Geometry check sheet. Reference: the model listing, model coordinates, mm. Give positions to 0.01 mm unless a question says otherwise; leave off trailing zeros. Loops run counter-clockwise (first coordinate to the right, second up) from the corner with the lowest first, then second, coordinate; pieces in that order, holes last.
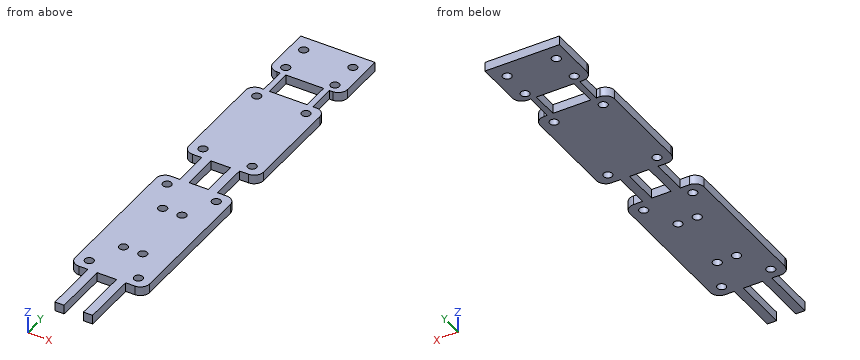
```python
from build123d import *

# Parameters (mm, degrees)
SKETCH1_R           = 0.95
SKETCH1_W           = 4.2
SKETCH1_H           = 8
SKETCH1_W_2         = 8.2
SKETCH1_H_2         = 6
BOSS_EXTRUDE1_DEPTH = 2


with BuildPart() as part:
    # Sketch1 → Boss-Extrude1 (new body)
    with BuildSketch(Plane.XY):
        with BuildLine():
            Line((16.2, 109.64), (0, 109.64))
            Line((0, 109.64), (0, 99.66))
            ThreePointArc((0, 99.66), (0.585786438, 98.245786438), (2, 97.66))
            Line((2, 97.66), (2.75, 97.66))
            Line((2.75, 97.66), (2.75, 91.66))
            Line((2.75, 91.66), (2, 91.66))
            ThreePointArc((2, 91.66), (0.585786438, 91.074213562), (0, 89.66))
            Line((0, 89.66), (0, 69.21))
            ThreePointArc((0, 69.21), (0.585786438, 67.795786438), (2, 67.21))
            Line((2, 67.21), (4, 67.21))
            Line((4, 67.21), (4, 59.21))
            Line((4, 59.21), (2, 59.21))
            ThreePointArc((2, 59.21), (0.585786438, 58.624213562), (0, 57.21))
            Line((0, 57.21), (0, 28))
            ThreePointArc((0, 28), (0.585786438, 26.585786438), (2, 26))
            Line((2, 26), (4, 26))
            Line((4, 26), (4, 14))
            Line((4, 14), (6, 14))
            Line((6, 14), (6, 26))
            Line((6, 26), (10.2, 26))
            Line((10.2, 26), (10.2, 14))
            Line((10.2, 14), (12.2, 14))
            Line((12.2, 14), (12.2, 26))
            Line((12.2, 26), (14.2, 26))
            ThreePointArc((14.2, 26), (15.614213562, 26.585786438), (16.2, 28))
            Line((16.2, 28), (16.2, 57.21))
            ThreePointArc((16.2, 57.21), (15.614213562, 58.624213562), (14.2, 59.21))
            Line((14.2, 59.21), (12.2, 59.21))
            Line((12.2, 59.21), (12.2, 67.21))
            Line((12.2, 67.21), (14.2, 67.21))
            ThreePointArc((14.2, 67.21), (15.614213562, 67.795786438), (16.2, 69.21))
            Line((16.2, 69.21), (16.2, 89.66))
            ThreePointArc((16.2, 89.66), (15.614213562, 91.074213562), (14.2, 91.66))
            Line((14.2, 91.66), (13.45, 91.66))
            Line((13.45, 91.66), (13.45, 97.66))
            Line((13.45, 97.66), (14.2, 97.66))
            ThreePointArc((14.2, 97.66), (15.614213562, 98.245786438), (16.2, 99.66))
            Line((16.2, 99.66), (16.2, 109.64))
        make_face()
        with Locations((13.45, 56.71)):
            Circle(SKETCH1_R, mode=Mode.SUBTRACT)
        with Locations((10.2, 49.71)):
            Circle(SKETCH1_R, mode=Mode.SUBTRACT)
        with Locations((13.45, 106.16)):
            Circle(SKETCH1_R, mode=Mode.SUBTRACT)
        with Locations((2.75, 99.66)):
            Circle(SKETCH1_R, mode=Mode.SUBTRACT)
        with Locations((6, 49.71)):
            Circle(SKETCH1_R, mode=Mode.SUBTRACT)
        with Locations((2.75, 28.5)):
            Circle(SKETCH1_R, mode=Mode.SUBTRACT)
        with Locations((2.75, 89.16)):
            Circle(SKETCH1_R, mode=Mode.SUBTRACT)
        with Locations((2.75, 56.71)):
            Circle(SKETCH1_R, mode=Mode.SUBTRACT)
        with Locations((13.45, 89.16)):
            Circle(SKETCH1_R, mode=Mode.SUBTRACT)
        with Locations((13.45, 99.66)):
            Circle(SKETCH1_R, mode=Mode.SUBTRACT)
        with Locations((13.45, 69.71)):
            Circle(SKETCH1_R, mode=Mode.SUBTRACT)
        with Locations((6, 35.5)):
            Circle(SKETCH1_R, mode=Mode.SUBTRACT)
        with Locations((2.75, 106.16)):
            Circle(SKETCH1_R, mode=Mode.SUBTRACT)
        with Locations((10.2, 35.5)):
            Circle(SKETCH1_R, mode=Mode.SUBTRACT)
        with Locations((2.75, 69.71)):
            Circle(SKETCH1_R, mode=Mode.SUBTRACT)
        with Locations((13.45, 28.5)):
            Circle(SKETCH1_R, mode=Mode.SUBTRACT)
        with Locations((8.1, 63.21)):
            Rectangle(SKETCH1_W, SKETCH1_H, mode=Mode.SUBTRACT)
        with Locations((8.1, 94.66)):
            Rectangle(SKETCH1_W_2, SKETCH1_H_2, mode=Mode.SUBTRACT)
    extrude(amount=BOSS_EXTRUDE1_DEPTH)


solid = part.part
```
1) Sectioned sample at A-A on y = 96. Enter the section's corners in (x, z), plus the area to 3 significant figures.
2) Depth check by flat-ended pin: P1, Ø0.6, axis at y = 65, z = 1, coming from the -X side; P2, Ø0.6, axis at x = 7.5, z = 1, coming from the -Y side; P3, Ø1, axis at y = 63, z = 1, coming from the +X side. Enter the tip coordinate at first touch or a pass-through.
3) Scan lines: line 1 along Y through (x, z) = (8.5, 0.1); line 2 along X through (y, z) = (106.16, 1.35); line 3 along X through (y, z) = (63, 0.8). Record each from-to range of solid material in increasing order.
4) Sectioned sample at B-B on z = 1.65. Count the separate pieces of the cut face and the enclosed holes in it, plus the area to 3 significant figures.
Determined:
1. outline: (2.75, 0) - (4, 0) - (4, 2) - (2.75, 2) - close; (12.2, 0) - (13.45, 0) - (13.45, 2) - (12.2, 2) - close
1. area: 5.00 mm2
2. P1: stops at x = 4
2. P2: stops at y = 26
2. P3: stops at x = 12.2
3. line 1: y = 26 to 59.21, 67.21 to 91.66, 97.66 to 109.64
3. line 2: x = 0 to 1.8, 3.7 to 12.5, 14.4 to 16.2
3. line 3: x = 4 to 6, 10.2 to 12.2
4. separate pieces: 1
4. enclosed holes: 18
4. area: 1,170 mm2
